Part model, mm, in its own coordinate system. Face numbers are marked on the shaded views. A direction names the side the tool comes from. Round coordinates to 2 decimals unless told otherwise and drop trailing zeros. Write each loop counter-clockwise with the first axis right and the second up, starting at its lowest first coordinate (ties: lowest second). Pieces come first, ordered by that corner, then holes. Notation, with made-up numbers: (-31, -17) -> (12, -17) arc R31 cw to (12, 9) -> close; hole circle Ø2 at (-25, 32). An arc over 180 degrees is marked (long way). Return JSON: item names as keys, results as strings. Group by question number.
(1) Saw through at D-D (x = 5.5). List the corners of the cut face in (y, z).
(2) Saw through at C-C (z = 3.5). List the corners of the cut face in (x, y).
(3) Drill centre lines: L1, parallel to Y at x = 0, z = 12.85; L2, parallel to Y at x = 0, z = 6.25; L3, parallel to X at y = -0.25, z = 15. Where is each one in solid material? Low to high. Write a range as from..to.
(4) Drop flat-ended pins along their axis: pin 1 Ø5 at (x, z) = (-6.5, 3) entering from +Y; pin 2 Ø5 at (y, z) = (-5.5, 12) entering from -X; pin 3 Ø6 at (x, z) = (2, 6.5) entering from +Y. Give the stop position or say it passes through.
(5) Tool access for the marked faces 1 and 2: list every direction of +Z, -Z, +X, -X, +Y, -Y with a clear straight run to the whole face (end or side of a thin tool).
(6) Saw through at A-A (y = 0). List the corners of the cut face in (x, z), plus the area to 3 significant figures.
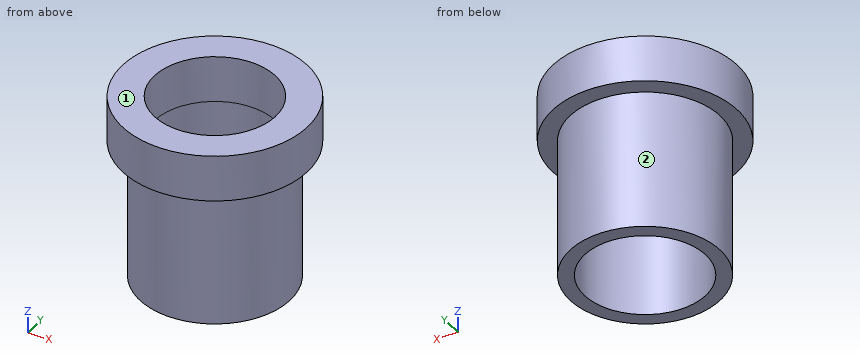
from build123d import *

# Parameters (mm, degrees)
SKETCH1_R           = 6.5
BOSS_EXTRUDE1_DEPTH = 12
SKETCH2_R           = 5.25
CUT_EXTRUDE1_DEPTH  = 14
SKETCH4_R           = 8
BOSS_EXTRUDE2_DEPTH = 4
SKETCH5_R           = 5.25
CUT_EXTRUDE2_DEPTH  = 17.492422502


with BuildPart() as part:
    # Sketch1 → Boss-Extrude1 (new body)
    with BuildSketch(Plane.XY):
        Circle(SKETCH1_R)
    extrude(amount=BOSS_EXTRUDE1_DEPTH)

    # Sketch2 → Cut-Extrude1 (cut)
    with BuildSketch(Plane.XY):
        Circle(SKETCH2_R)
    extrude(amount=CUT_EXTRUDE1_DEPTH, mode=Mode.SUBTRACT)

    # Sketch4 → Boss-Extrude2 (add)
    with BuildSketch(Plane.XY.offset(12)):
        Circle(SKETCH4_R)
    extrude(amount=BOSS_EXTRUDE2_DEPTH)

    # Sketch5 → Cut-Extrude2 (cut, through all)
    with BuildSketch(Plane(origin=(0, 0, 12), x_dir=(-1, 0, 0), z_dir=(0, 0, -1))):
        Circle(SKETCH5_R)
    extrude(amount=-CUT_EXTRUDE2_DEPTH, mode=Mode.SUBTRACT)


solid = part.part
Computed values:
{
 "1": {"outline": "(-5.81, 12) -> (-3.46, 12) -> (-3.46, 0) -> (3.46, 0) -> (3.46, 12) -> (5.81, 12) -> (5.81, 16) -> (-5.81, 16) -> close"},
 "2": {"outline": "circle Ø13 at (0, 0); hole circle Ø10.5 at (0, 0)"},
 "3": {"L1": "-8..-5.25, 5.25..8", "L2": "-6.5..-5.25, 5.25..6.5", "L3": "-8..-5.24, 5.24..8"},
 "4": {"pin 1": "y = 5.12", "pin 2": "x = -7.42", "pin 3": "y = 6.5"},
 "5": {"face 1": "+Z, +X, -X, +Y, -Y", "face 2": "-Z"},
 "6": {"outline": "(-8, 12) -> (-6.5, 12) -> (-6.5, 0) -> (-5.25, 0) -> (-5.25, 16) -> (-8, 16) -> close; (5.25, 0) -> (6.5, 0) -> (6.5, 12) -> (8, 12) -> (8, 16) -> (5.25, 16) -> close", "area": "52.0 mm2"}
}
